CAD build for the part. Positions are in the model's coordinates, mm. Round coordinates to 2 decimals unless told otherwise and drop trailing zeros. Write each loop counter-clockwise with the first axis right and the second up, starting at its lowest first coordinate (ties: lowest second). Pieces come first, ordered by that corner, then holes. Notation, with made-up numbers: (89.25, 75) - (123.25, 75) arc R16 ccw to (123.25, 86) - close; hole circle Ø1 at (-18, 18). An arc over 180 degrees is marked (long way). Put each result on its own line as item: value. Start each with the question number.
Item 1: Cut at C-C (x = 311). Give the cut face in (y, z) (3 decimals).
Item 2: Drill centre lines: line 1 (Z direction, x = 166, y = -2) (3 decimals); line 2 (Y direction, x = 364, z = 2.5) (3 decimals); line 3 (X direction, y = 0.25, z = 2.25). Where is each one in solid material? Low to high. Write a range as from..to.
Item 3: Pin check, flat tip, straight feed: pin 1 Ø1 at (x, y) = (290.5, 1.5) entering from -Z. Stop position of the tip, or through.
Item 4: Cut at A-A (y = 0). Give the cut face in (x, z) (3 decimals), and give its area (3 significant figures).
Item 5: Cut at B-B (z = -2). Give the cut face in (x, y) (3 decimals).
Autodesk Inventor part; units mm, degrees
ref_plane "YZ Plane" through (0, 0, 0) normal (1, 0, 0) x (0, 1, 0)
ref_plane "XZ Plane" through (0, 0, 0) normal (0, 1, 0) x (-1, 0, 0)
ref_plane "XY Plane" through (0, 0, 0) normal (0, 0, 1) x (1, 0, 0)
sketch "Boceto1" plane through (0, 0, 0) normal (0, 0, 1) x (1, 0, 0)
  arc A0 (0, 3.175) -> (0, -3.175) centre (0, 0) ccw
  line L0 (360.825, 0) -> (364, 0)
  arc A1 (364, -3.175) -> (364, 3.175) centre (364, 0) ccw
  line L1 (0, 3.175) -> (364, 3.175)
  line L2 (364, -3.175) -> (0, -3.175)
  dimension "d0" = 6.35
  dimension "d1" = 364
  dimension "d2" = 6.35
extrude "Extrusión1" add sketch "Boceto1" along normal blind 3.175
sketch "Boceto2" plane through (0, 0, 0) normal (0, 0, -1) x (-1, 0, 0)
  circle A0 centre (0, 0) radius 2.675
  dimension "d5" = 5.35
extrude "Extrusión2" add sketch "Boceto2" along normal blind 3.175
sketch "Boceto3" plane through (0, 0, 0) normal (0, 0, -1) x (-1, 0, 0)
  arc A0 (-364, 3.175) -> (-364, -3.175) centre (-364, 0) ccw
  circle A1 centre (-364, 0) radius 2.675
  point P0 (0, 0)
  dimension "d8" = 5.35
extrude "Extrusión3" cut sketch "Boceto3" against normal blind 3.175
properties part number "eslasbon_2" material "Plástico ABS"
Output values:
1. outline: (-3.175, 0) - (3.175, 0) - (3.175, 3.175) - (-3.175, 3.175) - close
2. line 1: 0..3.175
2. line 2: -3.175..-2.675, 2.675..3.175
2. line 3: -3.17..361.34, 366.66..367.17
3. pin 1: z = 0
4. outline: (-3.175, 0) - (-2.675, 0) - (-2.675, -3.175) - (2.675, -3.175) - (2.675, 0) - (361.325, 0) - (361.325, 3.175) - (-3.175, 3.175) - close; (366.675, 0) - (367.175, 0) - (367.175, 3.175) - (366.675, 3.175) - close
4. area: 1,180 mm2
5. outline: circle Ø5.35 at (0, 0)
